Can you work these out from the model? Positions are in its coordinate system, mm. Round coordinates to 2 decimals unless told otherwise and drop trailing zeros. Order: outer loops, then holes, each group sorted by start corner. A loop starts at its lowest first (then second) coordinate and runs counter-clockwise, first axis right, second up. Notation, with made-up numbers: (-24, -22) - (-12, -22) arc R20 ccw to (-12, -11) - close; hole circle Ø1 at (-30, 10.25). An arc over 180 degrees is marked (long way). Write item = value, one per line.
from build123d import *

# Parameters (mm, degrees)
BOSS_EXTRUDE1_DEPTH      = 9.1948
BOSS_EXTRUDE1_DEPTH_BACK = 9.1948
SKETCH3_R                = 5.588
SKETCH4_OUTSIDE_W        = 25.942
SKETCH4_OUTSIDE_H        = 28.644
SKETCH4_OUTSIDE_R        = 8.73125
CUT_EXTRUDE1_DEPTH       = 3.9624
SKETCH5_OUTSIDE_W        = 25.942
SKETCH5_OUTSIDE_H        = 28.644
SKETCH5_OUTSIDE_R        = 8.73125
CUT_EXTRUDE2_DEPTH       = 3.0734
SKETCH6_OUTSIDE_W        = 180.058
SKETCH6_OUTSIDE_H        = 182.76
SKETCH6_OUTSIDE_R        = 8.73125
CUT_EXTRUDE3_DEPTH       = 20.647522197
CUT_EXTRUDE3_DRAFT       = -75
SKETCH7_OUTSIDE_W        = 184.996
SKETCH7_OUTSIDE_H        = 187.698
SKETCH7_OUTSIDE_R        = 8.73125
CUT_EXTRUDE4_DEPTH       = 21.309283864
CUT_EXTRUDE4_DRAFT       = -75
SKETCH8_R                = 7.14375
CUT_EXTRUDE5_DEPTH       = 14.4272
CHAMFER1_SIZE            = 0.381
FILLET1_R                = 0.508


with BuildPart() as part:
    # Sketch3 → Boss-Extrude1 (new, two sides: drawn at the far end of the back side and taken through both)
    with BuildSketch(Plane(origin=(0, 0, 0), x_dir=(0, 0, -1), z_dir=(1, 0, 0)).offset(-BOSS_EXTRUDE1_DEPTH_BACK)):
        Polygon((8.73125, 5.040989538), (0, 10.081979076), (-8.73125, 5.040989538), (-8.73125, -5.040989538), (0, -10.081979076), (8.73125, -5.040989538), align=None)
        Circle(SKETCH3_R, mode=Mode.SUBTRACT)
    extrude(amount=BOSS_EXTRUDE1_DEPTH + BOSS_EXTRUDE1_DEPTH_BACK)

    # Sketch4 outside → Cut-Extrude1 (cut)
    with BuildSketch(Plane.ZY.offset(9.1948)):
        Rectangle(SKETCH4_OUTSIDE_W, SKETCH4_OUTSIDE_H)
        with Locations(Location((0, 0, 0), (0, 0, 180))):
            Circle(SKETCH4_OUTSIDE_R, mode=Mode.SUBTRACT)
    extrude(amount=-CUT_EXTRUDE1_DEPTH, mode=Mode.SUBTRACT)

    # Sketch5 outside → Cut-Extrude2 (cut)
    with BuildSketch(Plane(origin=(9.1948, 0, 0), x_dir=(0, 0, -1), z_dir=(1, 0, 0))):
        Rectangle(SKETCH5_OUTSIDE_W, SKETCH5_OUTSIDE_H)
        Circle(SKETCH5_OUTSIDE_R, mode=Mode.SUBTRACT)
    extrude(amount=-CUT_EXTRUDE2_DEPTH, mode=Mode.SUBTRACT)


with BuildPart() as cut_extrude3_tool:
    # Sketch6 outside → Cut-Extrude3 (with draft: the straight prism first)
    with BuildSketch(Plane.ZY.offset(5.2324)):
        Rectangle(SKETCH6_OUTSIDE_W, SKETCH6_OUTSIDE_H)
        with Locations(Location((0, 0, 0), (0, 0, 180))):
            Circle(SKETCH6_OUTSIDE_R, mode=Mode.SUBTRACT)
    extrude(amount=-CUT_EXTRUDE3_DEPTH)
    # Cut-Extrude3: the draft: its side faces are tilted about the plane it starts from
    cut_extrude3_sides = [cut_extrude3_tool.faces().sort_by_distance(p)[0] for p in [
        (5.091361099, -91.38, 0),
        (5.091361099, 0, 90.029),
        (5.091361099, 91.38, 0),
        (5.091361099, 0, -90.029),
        (5.091361099, 0, 8.73125),
    ]]
    draft(cut_extrude3_sides, Plane.ZY.offset(5.2324), CUT_EXTRUDE3_DRAFT)


with BuildPart() as part_1:
    add(part.part)

    # Cut-Extrude3: cut by cut_extrude3_tool
    add(cut_extrude3_tool.part, mode=Mode.SUBTRACT)


with BuildPart() as cut_extrude4_tool:
    # Sketch7 outside → Cut-Extrude4 (with draft: the straight prism first)
    with BuildSketch(Plane(origin=(6.1214, 0, 0), x_dir=(0, 0, -1), z_dir=(1, 0, 0))):
        Rectangle(SKETCH7_OUTSIDE_W, SKETCH7_OUTSIDE_H)
        Circle(SKETCH7_OUTSIDE_R, mode=Mode.SUBTRACT)
    extrude(amount=-CUT_EXTRUDE4_DEPTH)
    # Cut-Extrude4: the draft: its side faces are tilted about the plane it starts from
    cut_extrude4_sides = [cut_extrude4_tool.faces().sort_by_distance(p)[0] for p in [
        (-4.533241932, -93.849, 0),
        (-4.533241932, 0, -92.498),
        (-4.533241932, 93.849, 0),
        (-4.533241932, 0, 92.498),
        (-4.533241932, 0, 8.73125),
    ]]
    draft(cut_extrude4_sides, Plane(origin=(6.1214, 0, 0), x_dir=(0, 0, -1), z_dir=(1, 0, 0)), CUT_EXTRUDE4_DRAFT)


with BuildPart() as part_2:
    add(part_1.part)

    # Cut-Extrude4: cut by cut_extrude4_tool
    add(cut_extrude4_tool.part, mode=Mode.SUBTRACT)

    # Sketch8 → Cut-Extrude5 (cut)
    with BuildSketch(Plane(origin=(9.1948, 0, 0), x_dir=(0, 0, -1), z_dir=(1, 0, 0))):
        Circle(SKETCH8_R)
    extrude(amount=-CUT_EXTRUDE5_DEPTH, mode=Mode.SUBTRACT)

    # Chamfer1
    chamfer1_edges = [part_2.edges().sort_by_distance(p)[0] for p in [
        (-9.1948, 0, 5.588),
        (-5.2324, 0, 5.588),
    ]]
    chamfer(chamfer1_edges, length=CHAMFER1_SIZE)

    # Fillet1
    fillet1_edges = [part_2.edges().sort_by_distance(p)[0] for p in [
        (-9.1948, 0, 8.73125),
        (9.1948, 0, 8.73125),
    ]]
    fillet(fillet1_edges, radius=FILLET1_R)


solid = part_2.part
(1) If I drill on line 1 (Y direction, x = -7.4, z = 0); line 2 (Z direction, x = -4.5, y = 3.5); line 3 (Y direction, x = -1.25, z = -3.5), over which ranges is the centre line in solid material (lowest first)? Write a range as from..to.
Computed:
line_1 = -8.73..-5.59, 5.59..8.73
line_2 = -8.73..-6.23, 6.23..8.73
line_3 = -8.06..-6.23, 6.23..8.06
(2) If we section it at A-A (x = -3): Write out the boundary of the cut face in (y, z).
Computed:
outline = (-10.08, 0) - (-5.04, -8.73) - (5.04, -8.73) - (10.08, 0) - (5.04, 8.73) - (-5.04, 8.73) - close; hole circle Ø14.29 at (0, 0)
(3) Will these pins go through, and if not, where does the flat tip stop? P1, Ø1, axis at x = -6.5, z = -5.5, coming from the -Y side; P2, Ø5, axis at y = 1, z = -5.5, coming from the -X side; P3, Ø1, axis at x = -7, y = 3, coming from the -Z side; P4, Ø1, axis at x = 4, z = -3.5, coming from the -Y side.
Computed:
P1 = -7.16
P2 = -9.19
P3 = -8.37
P4 = -8.35
(4) Thinking about a two-plate mould opening in Z: for faces 1 (the face through (-6.984, 8.524, 1.893)), 2 (the face through (2.082, 0.314, 7.137)), 3 (the face through (0, 0, 8.731)), which applies, +Z half, -Z half, draft (parallel to the pull), parting line (faces both ways), or undercut?
Computed:
face_1 = parting line
face_2 = undercut
face_3 = +Z half
